Source: CAD feature listing. Evaluate the final solid. Frame: model axes, mm. A direction names the side the tool comes from. Round coordinates to 2 decimals unless told otherwise and drop trailing zeros. Write each loop counter-clockwise with the first axis right and the second up, starting at its lowest first coordinate (ties: lowest second). Pieces come first, ordered by that corner, then holes. Notation, with made-up numbers: M -33,63 L -3,63 A25 cw -3,91 Z; hole C 27.25,85 d9. An arc over 180 degrees is marked long. Use a Markdown table: item, result.
Autodesk Fusion 360 part; units mm, degrees
sketch "スケッチ1" plane through (0, 0, 0) normal (0, 0, 1) x (1, 0, 0)
  line L0 (13.3028, 9.942) -> (65, 5.4191)
  line L1 (0, 125) -> (0, 0)
  line L2 (0, 0) -> (65, 0)
  line L3 (65, 5.4191) -> (65, 0)
  line L4 (6, 107.0884) -> (6, 17.9116)
  arc A0 (6, 17.9116) -> (13.3028, 9.942) centre (14, 17.9116) ccw
  line L5 (65, 119.5809) -> (13.3028, 115.058)
  line L6 (0, 125) -> (65, 125)
  arc A1 (13.3028, 115.058) -> (6, 107.0884) centre (14, 107.0884) ccw
  line L7 (65, 125) -> (65, 119.5809)
extrude "押し出し1" add sketch "スケッチ1" along normal blind 100
Q1. Section C-C on x = 9.5. Return loops of the section in (y, z).
Results are:
| item | result |
|---|---|
| outline | M 0,0 L 11.3,0 L 11.3,100 L 0,100 Z; M 113.7,0 L 125,0 L 125,100 L 113.7,100 Z |
Q2. Section A-A on x = 26. Return loops of the section in (y, z).
Results are:
| item | result |
|---|---|
| outline | M 0,0 L 8.83,0 L 8.83,100 L 0,100 Z; M 116.17,0 L 125,0 L 125,100 L 116.17,100 Z |
Q3. First-contact query: pin 1 Ø1 at (y, z) = (17, 69.5) entering from +X; pin 2 Ø8 at (y, z) = (44.5, 59.5) entering from +X. Flat tips, straight axial feed; report the tip coordinate or a pass-through.
Results are:
| item | result |
|---|---|
| pin 1 | x = 6.13 |
| pin 2 | x = 6 |
Q4. Line query: L1, parallel to X at y = 23.5, z = 26; L2, parallel to Y at x = 19.5, z = 72; L3, parallel to Y at x = 32.5, z = 84. Output: solid intervals per line, ascending.
Results are:
| item | result |
|---|---|
| L1 | 0 to 6 |
| L2 | 0 to 9.4, 115.6 to 125 |
| L3 | 0 to 8.26, 116.74 to 125 |
Q5. Mould query, pull axis Y, two halves, no side actions, for faces 3 (the flat face through (0, 63, 49)), 4 (the flat face through (32, 0, 49)), 5 (the cylindrical face through (8.046, 112.432, 49.3)), 6 (the flat face through (32, 125, 49)). Classes: +Y half, -Y half, draft (parallel to the pull), parting line (faces both ways), or undercut.
Results are:
| item | result |
|---|---|
| face 3 | draft |
| face 4 | -Y half |
| face 5 | undercut |
| face 6 | +Y half |
Q6. Reachability of faces 1 (the flat face through (6, 63, 49)), 2 (the flat face through (3, 72, 0)) from +Z, -Z, +X, -X, +Y, -Y: full face, straight path, thin tool, end or side. Return the list, or none.
Results are:
| item | result |
|---|---|
| face 1 | +Z, -Z, +X |
| face 2 | -Z, +X, -X, +Y, -Y |
Q7. Section B-B on z = 88.5. Return loops of the section in (x, y).
Results are:
| item | result |
|---|---|
| outline | M 0,0 L 65,0 L 65,5.42 L 13.3,9.94 A8 cw 6,17.91 L 6,107.09 A8 cw 13.3,115.06 L 65,119.58 L 65,125 L 0,125 Z |
Q8. Section D-D on y = 76.5. Return loops of the section in (x, z), plus the area to 3 significant figures.
Results are:
| item | result |
|---|---|
| outline | M 0,0 L 6,0 L 6,100 L 0,100 Z |
| area | 600 mm^2 |
